CAD build for the part. Positions are in the model's coordinates, mm. A direction names the side the tool comes from. Give positions to 0.01 mm unless a question says otherwise; leave off trailing zeros. Loops run counter-clockwise (first coordinate to the right, second up) from the corner with the lowest first, then second, coordinate; pieces in that order, holes last.
```python
from build123d import *

# Parameters (mm, degrees)
SKETCH1_W           = 30
SKETCH1_H           = 30
BOSS_EXTRUDE1_DEPTH = 50
SKETCH2_R           = 10
CUT_EXTRUDE1_DEPTH  = 31
SKETCH3_R           = 11.2
CUT_EXTRUDE2_DEPTH  = 7
SKETCH4_W           = 30
SKETCH4_H           = 30
BOSS_EXTRUDE2_DEPTH = 10
SKETCH5_R           = 4.1
CUT_EXTRUDE3_DEPTH  = 61
CUT_EXTRUDE4_START  = -20
CUT_EXTRUDE4_DEPTH  = 30


with BuildPart() as part:
    # Sketch1 → Boss-Extrude1 (new body)
    with BuildSketch(Plane(origin=(0, 0, 0), x_dir=(1, 0, 0), z_dir=(0, 1, 0))):
        Rectangle(SKETCH1_W, SKETCH1_H)
    extrude(amount=BOSS_EXTRUDE1_DEPTH)

    # Sketch2 → Cut-Extrude1 (cut, through all)
    with BuildSketch(Plane.XY.offset(15)):
        with Locations((0, 25)):
            Circle(SKETCH2_R)
    extrude(amount=-CUT_EXTRUDE1_DEPTH, mode=Mode.SUBTRACT)

    # Sketch3 → Cut-Extrude2 (cut)
    with BuildSketch(Plane.XY.offset(15)):
        with Locations((0, 25)):
            Circle(SKETCH3_R)
    extrude(amount=-CUT_EXTRUDE2_DEPTH, mode=Mode.SUBTRACT)

    # Sketch4 → Boss-Extrude2 (add)
    with BuildSketch(Plane(origin=(0, 50, 0), x_dir=(1, 0, 0), z_dir=(0, 1, 0))):
        Rectangle(SKETCH4_W, SKETCH4_H)
    extrude(amount=BOSS_EXTRUDE2_DEPTH)

    # Sketch5 → Cut-Extrude3 (cut, through all)
    with BuildSketch(Plane(origin=(0, 60, 0), x_dir=(1, 0, 0), z_dir=(0, 1, 0))):
        with Locations(Location((0, 0, 0), (0, 0, 270))):  # turned: the seam where the file's is
            Circle(SKETCH5_R)
    extrude(amount=-CUT_EXTRUDE3_DEPTH, mode=Mode.SUBTRACT)

    # Sketch6 → Cut-Extrude4 (cut)
    with BuildSketch(Plane(origin=(0, 60, 0), x_dir=(1, 0, 0), z_dir=(0, 1, 0)).offset(CUT_EXTRUDE4_START)):
        Polygon((-3.7, 6.408587988), (-7.4, 0), (-3.7, -6.408587988), (3.7, -6.408587988), (7.4, 0), (3.7, 6.408587988), align=None)
    extrude(amount=-CUT_EXTRUDE4_DEPTH, mode=Mode.SUBTRACT)


solid = part.part
```
1. Probe line 1 along X through (y, z) = (18, 0); line 2 along Z through (x, y) = (-3.5, 13.5); line 3 along X through (y, z) = (2.5, 0). List the from-to ranges inside material, lowest first.
Responses:
line 1: x = -15 to -7.4, 7.4 to 15
line 2: z = -15 to -6.41, 6.41 to 15
line 3: x = -15 to -4.1, 4.1 to 15
2. Saw through at D-D, the plane y = 11. List the corners of the cut face in (x, z).
Responses:
outline: (-15, -15) - (15, -15) - (15, 15) - (-15, 15) - close; hole (-7.4, 0) - (-3.7, -6.41) - (3.7, -6.41) - (7.4, 0) - (3.7, 6.41) - (-3.7, 6.41) - close
3. Saw through at B-B, the plane z = -8.5. List the corners of the cut face in (x, y).
Responses:
outline: (-15, 0) - (15, 0) - (15, 60) - (-15, 60) - close; hole circle Ø20 at (0, 25)
4. Saw through at C-C, the plane y = 25. List the corners of the cut face in (x, z).
Responses:
outline: (-15, -15) - (-10, -15) - (-10, 8) - (-11.2, 8) - (-11.2, 15) - (-15, 15) - close; (10, -15) - (15, -15) - (15, 15) - (11.2, 15) - (11.2, 8) - (10, 8) - close
5. Saw through at A-A, the plane x = 0. List the corners of the cut face in (y, z).
Responses:
outline: (0, -15) - (15, -15) - (15, -6.41) - (10, -6.41) - (10, -4.1) - (0, -4.1) - close; (0, 4.1) - (10, 4.1) - (10, 6.41) - (15, 6.41) - (15, 8) - (13.8, 8) - (13.8, 15) - (0, 15) - close; (35, -15) - (60, -15) - (60, -4.1) - (40, -4.1) - (40, -6.41) - (35, -6.41) - close; (35, 6.41) - (40, 6.41) - (40, 4.1) - (60, 4.1) - (60, 15) - (36.2, 15) - (36.2, 8) - (35, 8) - close
6. Tool access for faces 4 (the face through (0, 37, 6.409)), 5 (the face through (-7.37, 31.76, -3.34)), 6 (the face through (-2.428, 14.066, 11.549)): list every direction of +Z, -Z, +X, -X, +Y, -Y with a clear straight run to the whole face (end or side of a thin tool).
Responses:
face 4: none
face 5: +Z, -Z
face 6: +Z
7. Pull direction Z, two halves, no side cores. Call faces 1 (the face through (4.065, 5.07, -0.534)), 2 (the face through (3, 36, 15)), 3 (the face through (-4, 0, -4)): released by +Z, released by -Z, zero draft, split by the parting line, or undercut.
Responses:
face 1: undercut
face 2: released by +Z
face 3: zero draft
